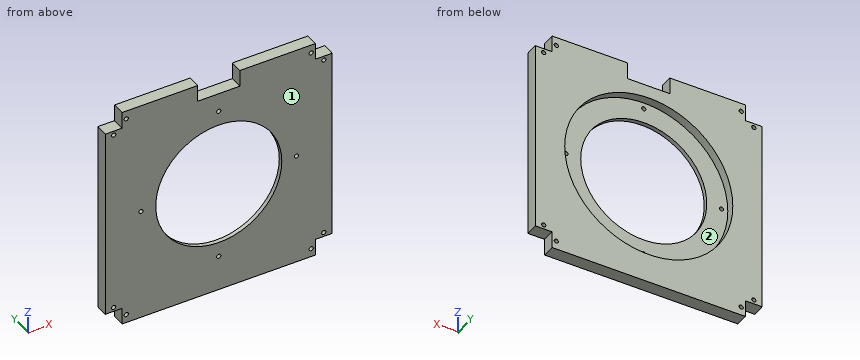
```python
from build123d import *

# Parameters (mm, degrees)
SKETCH1_W           = 270
SKETCH1_H           = 270
BOSS_EXTRUDE1_DEPTH = 15
SKETCH8_W           = 20
SKETCH8_H           = 20
CUT_EXTRUDE1_DEPTH  = 16
SKETCH9_R           = 2.5
CUT_EXTRUDE2_DEPTH  = 16
SKETCH10_R          = 100
CUT_EXTRUDE3_DEPTH  = 10
SKETCH12_R          = 75
SKETCH12_R_2        = 2.5
CUT_EXTRUDE4_DEPTH  = 6
SKETCH13_W          = 50
SKETCH13_H          = 20
CUT_EXTRUDE5_DEPTH  = 15


with BuildPart() as part:
    # Sketch1 → Boss-Extrude1 (new body)
    with BuildSketch(Plane(origin=(0, 0, 0), x_dir=(1, 0, 0), z_dir=(0, 1, 0))):
        with Locations((135, 135)):
            Rectangle(SKETCH1_W, SKETCH1_H)
    extrude(amount=BOSS_EXTRUDE1_DEPTH)

    # Sketch8 → Cut-Extrude1 (cut, through all)
    with BuildSketch(Plane(origin=(0, 15, 0), x_dir=(1, 0, 0), z_dir=(0, 1, 0))):
        with Locations((10, 260)):
            Rectangle(SKETCH8_W, SKETCH8_H)
        with Locations((260, 260)):
            Rectangle(SKETCH8_W, SKETCH8_H)
        with Locations((260, 10)):
            Rectangle(SKETCH8_W, SKETCH8_H)
        with Locations((10, 10)):
            Rectangle(SKETCH8_W, SKETCH8_H)
    extrude(amount=-CUT_EXTRUDE1_DEPTH, mode=Mode.SUBTRACT)

    # Sketch9 → Cut-Extrude2 (cut, through all)
    with BuildSketch(Plane(origin=(0, 15, 0), x_dir=(1, 0, 0), z_dir=(0, 1, 0))):
        with Locations((10, 245)):
            Circle(SKETCH9_R)
        with Locations((10, 25)):
            Circle(SKETCH9_R)
        with Locations((25, 10)):
            Circle(SKETCH9_R)
        with Locations((245, 10)):
            Circle(SKETCH9_R)
        with Locations((260, 25)):
            Circle(SKETCH9_R)
        with Locations((260, 245)):
            Circle(SKETCH9_R)
        with Locations((245, 260)):
            Circle(SKETCH9_R)
        with Locations((25, 260)):
            Circle(SKETCH9_R)
    extrude(amount=-CUT_EXTRUDE2_DEPTH, mode=Mode.SUBTRACT)

    # Sketch10 → Cut-Extrude3 (cut)
    with BuildSketch(Plane(origin=(0, 15, 0), x_dir=(1, 0, 0), z_dir=(0, 1, 0))):
        with Locations((135, 135)):
            Circle(SKETCH10_R)
    extrude(amount=-CUT_EXTRUDE3_DEPTH, mode=Mode.SUBTRACT)

    # Sketch12 → Cut-Extrude4 (cut, through all)
    with BuildSketch(Plane(origin=(0, 5, 0), x_dir=(1, 0, 0), z_dir=(0, 1, 0))):
        with Locations((135, 135)):
            Circle(SKETCH12_R)
        with Locations((135, 227.5)):
            Circle(SKETCH12_R_2)
        with Locations((227.5, 135)):
            Circle(SKETCH12_R_2)
        with Locations((135, 42.5)):
            Circle(SKETCH12_R_2)
        with Locations((42.5, 135)):
            Circle(SKETCH12_R_2)
    extrude(amount=-CUT_EXTRUDE4_DEPTH, mode=Mode.SUBTRACT)

    # Sketch13 → Cut-Extrude5 (cut)
    with BuildSketch(Plane(origin=(0, 15, 0), x_dir=(1, 0, 0), z_dir=(0, 1, 0))):
        with Locations((135, 10)):
            Rectangle(SKETCH13_W, SKETCH13_H)
    extrude(amount=-CUT_EXTRUDE5_DEPTH, mode=Mode.SUBTRACT)


solid = part.part
```
The model under review builds one solid part; all positions refer to its coordinate system, in mm. Face numbers are marked on the shaded views. Round coordinates to 2 decimals unless told otherwise and drop trailing zeros. Loops run counter-clockwise (first coordinate to the right, second up) from the corner with the lowest first, then second, coordinate; pieces in that order, holes last.
1) Consider section C-C on y = 11.5. Give the number of separate pieces and of enclosed holes in the cut face, then the cut area to 3 significant figures.
Values follow:
separate pieces: 1
enclosed holes: 9
area: 38,700 mm2
2) Consider section B-B on x = 80.5. State the section outline as (y, z) points, then the cut area to 3 significant figures.
Values follow:
outline: (0, -270) - (15, -270) - (15, -218.84) - (5, -218.84) - (5, -186.52) - (0, -186.52) - close; (0, -83.48) - (5, -83.48) - (5, -51.16) - (15, -51.16) - (15, 0) - (0, 0) - close
area: 1,860 mm2
3) Wall thickness on line 1 along Z through (x, y) = (260, 8.5); line 2 along X through (y, z) = (11.25, -10); line 3 along X through (y, z) = (6.25, -245): over which ranges is each line inside the solid? List them lowest first.
Values follow:
line 1: z = -250 to -247.5, -242.5 to -27.5, -22.5 to -20
line 2: x = 20 to 22.5, 27.5 to 110, 160 to 242.5, 247.5 to 250
line 3: x = 0 to 7.5, 12.5 to 257.5, 262.5 to 270
4) Clearance check with flat-ended pins moving along their axes: P1, Ø3, axis at x = 123.5, y = 12, coming from the +Z side; P2, Ø7.5, axis at x = 255.5, y = 5, coming from the -Z side. State where each tip first meets the part, or that it passes through.
Values follow:
P1: stops at z = -20
P2: stops at z = -250
5) Consider section A-A on z = -77. State the section outline as (x, y) points, then the cut area to 3 significant figures.
Values follow:
outline: (0, 0) - (87.45, 0) - (87.45, 5) - (53.54, 5) - (53.54, 15) - (0, 15) - close; (182.55, 0) - (270, 0) - (270, 15) - (216.46, 15) - (216.46, 5) - (182.55, 5) - close
area: 1,950 mm2
6) The part is to be moulded in two halves that separate along X. For the marked faces 1 and 2, say which applies: pulls with the +X half, pulls with the -X half, needs draft (parallel to the pull), parting line crosses it, or undercut.
Values follow:
face 1: needs draft
face 2: undercut
